```python
from build123d import *

# Parameters (mm, degrees)
F1_DEPTH = 7.62


# Not quite as in the source:
# - a feature names something its author has since deleted; it is built from what else it names


with BuildPart() as f1:
    # F0 (on Top) → F1 (new body)
    with BuildSketch(Plane.XY):
        with BuildLine():
            ThreePointArc((28.0726799719, -12.1853696085), (41.4217161306, -15.8764714027), (54.48557809, -20.4760919879))
            Line((54.48557809, -20.4760919879), (54.48557809, -17.9360919879))
            ThreePointArc((54.48557809, -17.9360919879), (51.4967288592, -16.763821011), (48.4891792987, -15.6403956202))
            ThreePointArc((48.4891792987, -15.6403956202), (44.8602983758, -14.3584600038), (41.2070755106, -13.1476345109))
            ThreePointArc((41.2070755106, -13.1476345109), (38.6048957608, -12.3330871208), (35.9916952796, -11.5546205858))
            ThreePointArc((35.9916952796, -11.5546205858), (31.733320464, -10.3696867585), (27.4494413676, -9.2805567694))
            ThreePointArc((27.4494413676, -9.2805567694), (23.9583783923, -8.4680969379), (20.4531163964, -7.7192645032))
            ThreePointArc((20.4531163964, -7.7192645032), (16.632517094, -6.9785468001), (12.7980359257, -6.3134183048))
            ThreePointArc((12.7980359257, -6.3134183048), (8.7921771864, -5.7014539178), (4.7745823593, -5.1719858311))
            ThreePointArc((4.7745823593, -5.1719858311), (2.3888765712, -4.897241097), (0, -4.6515878779))
            ThreePointArc((0, -4.6515878779), (-3.408711726, -4.3518848821), (-6.8221133026, -4.111412028))
            ThreePointArc((-6.8221133026, -4.111412028), (-10.4071482604, -3.922869598), (-13.9950228451, -3.7996630199))
            ThreePointArc((-13.9950228451, -3.7996630199), (-17.6605592517, -3.7413156735), (-21.3265467845, -3.7511630261))
            ThreePointArc((-21.3265467845, -3.7511630261), (-24.644831847, -3.8188928365), (-27.9615056934, -3.9424957507))
            ThreePointArc((-27.9615056934, -3.9424957507), (-43.2450696176, -5.2385218831), (-58.3815462887, -7.7192645032))
            ThreePointArc((-58.3815462887, -7.7192645032), (-63.1505292395, -8.7544721801), (-67.8924174044, -9.907446573))
            ThreePointArc((-67.8924174044, -9.907446573), (-73.5380139988, -11.4440807397), (-79.1355054029, -13.1476345109))
            ThreePointArc((-79.1355054029, -13.1476345109), (-81.4068857464, -13.8911431732), (-83.6690823894, -14.6621426181))
            ThreePointArc((-83.6690823894, -14.6621426181), (-86.1587803012, -15.5463139993), (-88.6364011403, -16.4637831816))
            ThreePointArc((-88.6364011403, -16.4637831816), (-89.8911745679, -16.9429103569), (-91.1426533968, -17.430578221))
            ThreePointArc((-91.1426533968, -17.430578221), (-92.6613427932, -18.0356268436), (-94.1749608987, -18.6532525791))
            ThreePointArc((-94.1749608987, -18.6532525791), (-95.4778611275, -19.1966804672), (-96.7768352111, -19.7494274307))
            Line((-96.7768352111, -19.7494274307), (-96.7768352111, -22.2894274307))
            ThreePointArc((-96.7768352111, -22.2894274307), (-71.0235394951, -13.4887335549), (-44.319003481, -8.239713722))
            ThreePointArc((-44.319003481, -8.239713722), (-43.2806848499, -8.1104188526), (-42.2417086499, -7.9865188972))
            ThreePointArc((-42.2417086499, -7.9865188972), (-26.5950201746, -6.7772498749), (-10.9016764341, -6.7896617958))
            ThreePointArc((-10.9016764341, -6.7896617958), (-6.4890042329, -7.0136625153), (-2.0823062052, -7.3343878974))
            ThreePointArc((-2.0823062052, -7.3343878974), (-1.2360355683, -7.4071155247), (-0.3900791081, -7.4834107816))
            ThreePointArc((-0.3900791081, -7.4834107816), (12.3943473899, -9.0773217505), (25.050742044, -11.4851812603))
            ThreePointArc((25.050742044, -11.4851812603), (26.5630587768, -11.8294586082), (28.0726799719, -12.1853696085))
        make_face()
        with BuildLine():
            ThreePointArc((-44.319003481, -8.239713722), (-32.5703828211, -34.4389737288), (-6.5546215011, -22.2894274307))
            ThreePointArc((-6.5546215011, -22.2894274307), (-6.0039890378, -14.307850149), (-2.0823062052, -7.3343878974))
            ThreePointArc((-2.0823062052, -7.3343878974), (-6.4890042329, -7.0136625153), (-10.9016764341, -6.7896617958))
            ThreePointArc((-10.9016764341, -6.7896617958), (-25.5859305121, -33.2005400837), (-42.2417086499, -7.9865188972))
            ThreePointArc((-42.2417086499, -7.9865188972), (-43.2806848499, -8.1104188526), (-44.319003481, -8.239713722))
        make_face()
        with BuildLine():
            ThreePointArc((-6.5546215011, -22.2894274307), (16.5208344464, -36.9835014795), (28.0726799719, -12.1853696085))
            ThreePointArc((28.0726799719, -12.1853696085), (26.5630587768, -11.8294586082), (25.050742044, -11.4851812603))
            ThreePointArc((25.050742044, -11.4851812603), (8.5004214133, -33.8325331942), (-0.3900791081, -7.4834107816))
            ThreePointArc((-0.3900791081, -7.4834107816), (-1.2360355683, -7.4071155247), (-2.0823062052, -7.3343878974))
            ThreePointArc((-2.0823062052, -7.3343878974), (-6.0039890378, -14.307850149), (-6.5546215011, -22.2894274307))
        make_face()
    extrude(amount=F1_DEPTH)


solid = f1.part
```
Here's how the part is built. I have some questions about the finished solid (model axes, mm). A direction names the side the tool comes from. Coordinates: 2 decimals unless noted, no trailing zeros. Order: outer loops, then holes, each group sorted by start corner. A loop starts at its lowest first (then second) coordinate and runs counter-clockwise, first axis right, second up. Notation, with made-up numbers: M 81.5,30.5 L 104.5,30.5 A9 cw 104.5,46.5 Z; hole C 14.5,87.25 d11. An arc over 180 degrees is marked long. Answer as a JSON object with one key per item and string values. Group by question number.
(1) I need wall thicknesses on probe 1 along X at (y, z) = (-28, 5); probe 2 along X at (y, z) = (-24, 0.75); probe 3 along Y at (x, z) = (-20, 3.5). Which ranges of each line are inside material? Lowest first, please.
(2) If we mould it in two halves opening along Y, with no side actions, what happens to faces 1 (the face through (54.486, -19, 4)), 2 (the face through (-25.079, -33.174, 3.757))? For each: released by +Y, released by -Y, zero draft, split by the parting line, or undercut.
(3) Which directions (+Z, -Z, +X, -X, +Y, -Y) give clear straight access to the entire face, cutting with the end or side of a thin tool? Please do faces 3 (the face through (-96.777, -21, 4)), 4 (the face through (-26.815, -6.786, 3.757)).
(4) Suppose I cut it at A-A, the plane z = 3.75. Please give me the cut outline in (x, y), then the cut area to 3 significant figures.
(5) For pin 1 (4 mm diameter, centred on x = 28, z = 2.5, fed in from +Y), with a flat end and sliding along its axis, tell me the tip position at first contact or that it passes through.
(6) Suppose I cut it at C-C, the plane y = -31.5. Please give me the cut outline in (x, z), then the cut area to 3 significant figures.
(7) Suppose I cut it at B-B, the plane x = 3. Please give me the cut outline in (y, z).
(8) Suppose I cut it at D-D, the plane x = -37. Please give me the cut outline in (y, z), then the cut area to 3 significant figures.
Values found:
{
 "1": {"probe 1": "x = -41.39 to -38.8, -13.73 to -9.7, -4.67 to -1.42, 23.3 to 27.52", "probe 2": "x = -43.84 to -41.78, -10.74 to -7.25, -6.21 to -3.69, 25.57 to 29.06", "probe 3": "y = -34.93 to -32.07, -6.63 to -3.74"},
 "2": {"face 1": "zero draft", "face 2": "undercut"},
 "3": {"face 3": "+Z, -Z, -X, +Y, -Y", "face 4": "+Z, -Z"},
 "4": {"outline": "M -96.78,-22.29 A201.45 cw -44.32,-8.24 A20.15 ccw long -6.55,-22.29 A18.19 ccw long 28.07,-12.19 A201.45 cw 54.49,-20.48 L 54.49,-17.94 A197.07 ccw -88.64,-16.46 A197.07 ccw -91.14,-17.43 A197.07 ccw -96.78,-19.75 Z; hole M -42.24,-7.99 A17.68 ccw long -10.9,-6.79 A201.45 ccw Z; hole M -0.39,-7.48 A15.69 ccw long 25.05,-11.49 A201.45 ccw Z", "area": "830 mm^2"},
 "5": {"pin 1": "stops at y = -8.94"},
 "6": {"outline": "M -37.86,0 L -33.85,0 L -33.85,7.62 L -37.86,7.62 Z; M -18.67,0 L -13.23,0 L -13.23,7.62 L -18.67,7.62 Z; M -2.27,0 L 2.41,0 L 2.41,7.62 L -2.27,7.62 Z; M 19.47,0 L 25.12,0 L 25.12,7.62 L 19.47,7.62 Z", "area": "151 mm^2"},
 "7": {"outline": "M -35.64,0 L -31.87,0 L -31.87,7.62 L -35.64,7.62 Z; M -7.83,0 L -4.96,0 L -4.96,7.62 L -7.83,7.62 Z"},
 "8": {"outline": "M -32.13,0 L -29.58,0 L -29.58,7.62 L -32.13,7.62 Z; M -7.44,0 L -4.56,0 L -4.56,7.62 L -7.44,7.62 Z", "area": "41.4 mm^2"}
}
